from build123d import *

# Parameters (mm, degrees)
BOSS_EXTRUDE1_DEPTH         = 34.625
BOSS_EXTRUDE2_DEPTH         = 0.85
BOSS_EXTRUDE3_DEPTH         = 1.3
LPATTERN1_COUNT             = 8
LPATTERN1_PITCH             = 9.5
M3_5X0_6_TAPPED_HOLE1_D     = 2.9
M3_5X0_6_TAPPED_HOLE1_DEPTH = 8
M3_5X0_6_TAPPED_HOLE1_TIP   = 0.871247898


with BuildPart() as part:
    # Sketch1 → Boss-Extrude1 (new body, symmetric)
    with BuildSketch(Plane(origin=(0, 0, 0), x_dir=(0, 0, -1), z_dir=(1, 0, 0))):
        Polygon((6.75, 0), (6.75, 2.79), (5.365, 9.1), (-5.365, 9.1), (-6.75, 2.79), (-6.75, 0), align=None)
    extrude(amount=BOSS_EXTRUDE1_DEPTH, both=True)

    # Sketch3 → Boss-Extrude2 (add)
    with BuildSketch(Plane(origin=(34.625, 0, 0), x_dir=(0, 0, -1), z_dir=(1, 0, 0))):
        with BuildLine():
            Line((-6.75, 0), (-7.35, 0))
            Line((-7.35, 0), (-7.35, 18.1))
            ThreePointArc((-7.35, 18.1), (-7.203553391, 18.453553391), (-6.85, 18.6))
            Line((-6.85, 18.6), (6.85, 18.6))
            ThreePointArc((6.85, 18.6), (7.203553391, 18.453553391), (7.35, 18.1))
            Line((7.35, 18.1), (7.35, 0))
            Line((7.35, 0), (6.75, 0))
            Line((6.75, 0), (6.75, 2.79))
            Line((6.75, 2.79), (5.365, 9.1))
            Line((5.365, 9.1), (-5.365, 9.1))
            Line((-5.365, 9.1), (-6.75, 2.79))
            Line((-6.75, 2.79), (-6.75, 0))
        make_face()
    boss_extrude2 = extrude(amount=-BOSS_EXTRUDE2_DEPTH)

    # Mirror1: Boss-Extrude2 across plane
    add(boss_extrude2.mirror(Plane(origin=(0, 0, 0), x_dir=(0, 0, 1), z_dir=(1, 0, 0))))

    # Sketch4 → Boss-Extrude3 (add)
    with BuildSketch(Plane.ZY.offset(-33.775)):
        with BuildLine():
            Line((7.35, 0), (7.35, 12.42))
            Line((7.35, 12.42), (4.588898397, 15.03))
            Line((4.588898397, 15.03), (6.438355915, 16.98652878))
            ThreePointArc((6.438355915, 16.98652878), (6.534203446, 17.527818591), (6.075, 17.83))
            Line((6.075, 17.83), (-6.075, 17.83))
            ThreePointArc((-6.075, 17.83), (-6.534203446, 17.527818591), (-6.438355915, 16.98652878))
            Line((-6.438355915, 16.98652878), (-4.588898397, 15.03))
            Line((-4.588898397, 15.03), (-7.35, 12.42))
            Line((-7.35, 12.42), (-7.35, 0))
            Line((-7.35, 0), (-6.75, 0))
            Line((-6.75, 0), (-6.75, 2.79))
            Line((-6.75, 2.79), (-5.365, 9.1))
            Line((-5.365, 9.1), (5.365, 9.1))
            Line((5.365, 9.1), (6.75, 2.79))
            Line((6.75, 2.79), (6.75, 0))
            Line((6.75, 0), (7.35, 0))
        make_face()
    boss_extrude3 = extrude(amount=BOSS_EXTRUDE3_DEPTH)

    # LPattern1: Boss-Extrude3 ×8
    with Locations(*[(-i * LPATTERN1_PITCH, 0, 0) for i in range(1, LPATTERN1_COUNT)]):
        add(boss_extrude3)

    # M3.5x0.6 Tapped Hole1
    with Locations(Plane(origin=(0, 9.1, 0), x_dir=(1, 0, 0), z_dir=(0, 1, 0))):
        with Locations((-28.625, 0), (-19.125, 0), (0, 0), (-0.125, 0), (9.375, 0), (18.875, 0), (28.375, 0), (-9.625, 0)):
            Hole(M3_5X0_6_TAPPED_HOLE1_D / 2, depth=M3_5X0_6_TAPPED_HOLE1_DEPTH)
            with Locations((0, 0, -(M3_5X0_6_TAPPED_HOLE1_DEPTH + M3_5X0_6_TAPPED_HOLE1_TIP / 2))):  # 118° drill point
                Cone(0, M3_5X0_6_TAPPED_HOLE1_D / 2, M3_5X0_6_TAPPED_HOLE1_TIP, mode=Mode.SUBTRACT)


solid = part.part
The model under review builds one solid part; all positions refer to its coordinate system, in mm. A direction names the side the tool comes from. Round coordinates to 2 decimals unless told otherwise and drop trailing zeros. Loops run counter-clockwise (first coordinate to the right, second up) from the corner with the lowest first, then second, coordinate; pieces in that order, holes last. Notation, with made-up numbers: M -37,-15 L 19,-15 A14 cw 19,1 Z; hole C 54.5,-18.5 d4. An arc over 180 degrees is marked long. Answer as CSV lines item,"result".
1. We need section A-A (y = 11.5). Count the separate pieces of the cut face and the enclosed holes in it, plus the area to 3 significant figures.
Outcome:
separate pieces,"8"
enclosed holes,"0"
area,"174 mm2"
2. To check wall thickness, follow L1, parallel to Y at x = -20.5, z = -2.75; L2, parallel to Z at x = -18, y = 7.75; L3, parallel to Z at x = -31, y = 1.25. State the ranges of each line that lie inside material, in increasing order. Write a range as [from, to].
Outcome:
L1,"y = [0, 9.1]"
L2,"z = [-5.66, -0.91], [0.91, 5.66]"
L3,"z = [-6.75, 6.75]"
3. Insertion check: pin 1 Ø4 at (x, z) = (-30.5, -1) entering from +Y; pin 2 Ø1 at (x, z) = (-4.5, 3) entering from +Y; pin 3 Ø3 at (x, y) = (26.5, 1) entering from +Z. Each pin has a flat end and moves straight along its axis. Give the tip position at first contact, or say it passes through.
Outcome:
pin 1,"stops at y = 9.1"
pin 2,"stops at y = 17.83"
pin 3,"stops at z = 6.75"
4. We need section B-B (x = -3). Give the boundary of the cut face in (y, z) (3 decimals).
Outcome:
outline,"M 0,-6.75 L 2.79,-6.75 L 9.1,-5.365 L 9.1,5.365 L 2.79,6.75 L 0,6.75 Z"
5. Draft analysis for pull direction Y (two halves, no side actions). For faces 5 (the face through (13.475, 13, 0)), 6 (the face through (23.634, 15.995, 5.501)), 7 (the face through (-27, 9.1, 0)), 8 (the face through (-14.366, 13.707, 5.989)), state which applies: pulls with the +Y half, pulls with the -Y half, needs draft (parallel to the pull), parting line crosses it, or undercut.
Outcome:
face 5,"needs draft"
face 6,"undercut"
face 7,"pulls with the +Y half"
face 8,"undercut"
6. For faces 1 (the face through (33.134, 13.707, 5.989)), 2 (the face through (17.492, 5.044, -0.436)), 3 (the face through (-8, 9.1, 0)), 4 (the face through (-10, 1, -6.75)), list the 3-axis set-ups (+Z, -Z, +X, -X, +Y, -Y) from which the entire face can be reached by the end or side of a thin tool; tool diameter is ignored.
Outcome:
face 1,"+Z"
face 2,"+Y"
face 3,"+Z, -Z, +Y"
face 4,"-Z, +Y, -Y"
